Geometry: final body of the model. Coordinates: model frame, mm. Face numbers are marked on the shaded views. A direction names the side the tool comes from. Give positions to 0.01 mm unless a question says otherwise; leave off trailing zeros. Write each loop counter-clockwise with the first axis right and the second up, starting at its lowest first coordinate (ties: lowest second). Pieces come first, ordered by that corner, then holes.
Q1. Cut plane B-B on x = -10.5. Return the cut outline in (y, z), plus the area to 3 significant figures.
Q2. Draft query along X for the marked faces 1, 2 and 3. Return one class per face: pulls with the +X half, pulls with the -X half, needs draft (parallel to the pull), parting line crosses it, or undercut.
Q3. Cut plane A-A on z = 0.6. Return the cut outline in (x, y).
Q4. Reachability of the marked faces 4 and 5 from +Z, -Z, +X, -X, +Y, -Y: full face, straight path, thin tool, end or side. Return the list, or none.
Q5. Line query: L1, parallel to X at y = -16, z = 4.45; L2, parallel to Z at x = -3, y = -18. Output: solid intervals per line, ascending.
Autodesk Inventor part; units mm, degrees
ref_plane "YZ Plane" through (0, 0, 0) normal (1, 0, 0) x (0, 1, 0)
ref_plane "XZ Plane" through (0, 0, 0) normal (0, 1, 0) x (-1, 0, 0)
ref_plane "XY Plane" through (0, 0, 0) normal (0, 0, 1) x (1, 0, 0)
sketch "스케치1" plane through (0, 0, 0) normal (0, 0, 1) x (1, 0, 0)
  line L0 (25, 25) -> (-25, 25)
  line L1 (-25, 25) -> (-25, -25)
  line L2 (-25, -25) -> (25, -25)
  line L3 (25, -25) -> (25, 25)
  line L4 (-23, 23) -> (23, 23)
  line L5 (23, 23) -> (23, -23)
  line L6 (23, -23) -> (-23, -23)
  line L7 (-23, -23) -> (-23, 23)
  point P0 (0, 0)
  dimension "d0" = 2
extrude "돌출1" add sketch "스케치1" along normal blind 5
sketch "스케치2" plane through (0, 0, 5) normal (0, 0, 1) x (1, 0, 0)
  line L0 (25, 25) -> (-25, 25)
  line L1 (-25, 25) -> (-25, -25)
  line L2 (-25, -25) -> (25, -25)
  line L3 (25, -25) -> (25, 25)
  point P0 (0, 0)
extrude "돌출2" add sketch "스케치2" along normal blind 1
properties part number "light box_3D 인쇄"
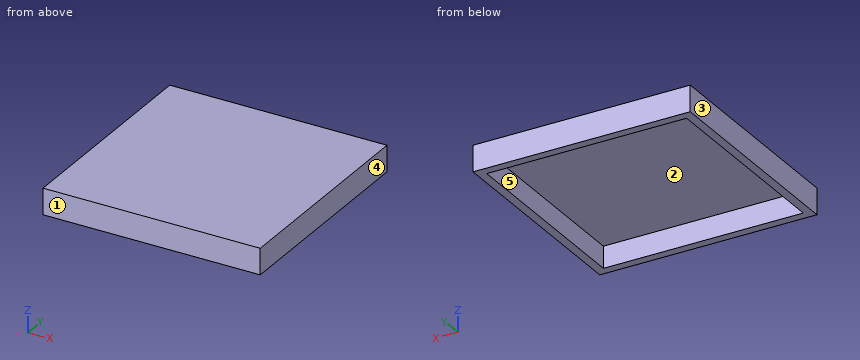
Data:
1. outline: (-25, 0) - (-23, 0) - (-23, 5) - (23, 5) - (23, 0) - (25, 0) - (25, 6) - (-25, 6) - close
1. area: 70.0 mm2
2. face 1: needs draft
2. face 2: undercut
2. face 3: pulls with the -X half
3. outline: (-25, -25) - (25, -25) - (25, 25) - (-25, 25) - close; hole (-23, -23) - (23, -23) - (23, 23) - (-23, 23) - close
4. face 4: +Z, -Z, +X, +Y, -Y
4. face 5: -Z
5. L1: x = -25 to -23, 23 to 25
5. L2: z = 5 to 6
